The model under review builds one solid part; all positions refer to its coordinate system, in mm. Round coordinates to 2 decimals unless told otherwise and drop trailing zeros. Order: outer loops, then holes, each group sorted by start corner. A loop starts at its lowest first (then second) coordinate and runs counter-clockwise, first axis right, second up.
from build123d import *

# Parameters (mm, degrees)
F0_W     = 20
F0_H     = 20
F1_DEPTH = 240
F2_R     = 2.5
F3_DEPTH = 25
F4_R     = 2.5
F5_DEPTH = 25


with BuildPart() as f1:
    # F0 (on Front) → F1 (new body)
    with BuildSketch(Plane.XZ):
        with Locations((24.677172, -22.298429)):
            Rectangle(F0_W, F0_H)
    extrude(amount=F1_DEPTH)

    # F2 (on face) → F3 (cut)
    with BuildSketch(Plane.XY.offset(-12.298429)):
        with Locations((24.677172, -230)):
            Circle(F2_R)
    extrude(amount=-F3_DEPTH, mode=Mode.SUBTRACT)

    # F4 (on face) → F5 (cut)
    with BuildSketch(Plane.XY.offset(-12.298429)):
        with Locations((24.677172, -10)):
            Circle(F4_R)
    extrude(amount=-F5_DEPTH, mode=Mode.SUBTRACT)


solid = f1.part
(1) We need section A-A (y = -10). Give the boundary of the cut face in (x, z), and give its area (3 significant figures).
(2) The part is to be moulded in two halves that separate along Y. For faces 1 (the cylindrical face through (22.69, -11.52, -22.16)), 2 (the flat face through (25, -240, -22)), 3 (the flat face through (34.677, -118, -22)), say which applies: pulls with the +Y half, pulls with the -Y half, needs draft (parallel to the pull), parting line crosses it, or undercut.
(3) We need section B-B (x = 24.5). Give the boundary of the cut face in (y, z), and give its area (3 significant figures).
(4) Clearance check with flat-ended pins moving along their axes: P1, Ø3, axis at x = 24.68, y = -10, coming from the -Z side; P2, Ø5, axis at x = 21, z = -28, coming from the +Y side. State where each tip first meets the part, or that it passes through.
(5) To check wall thickness, follow L1, parallel to Y at x = 24.25, z = -22.25; L2, parallel to X at y = -230, z = -22.75; L3, parallel to Y at x = 26.75, z = -23.75. State the ranges of each line that lie inside material, in increasing order.
Verdict:
1. outline: (14.68, -32.3) - (22.18, -32.3) - (22.18, -12.3) - (14.68, -12.3) - close; (27.18, -32.3) - (34.68, -32.3) - (34.68, -12.3) - (27.18, -12.3) - close
1. area: 300 mm2
2. face 1: undercut
2. face 2: pulls with the -Y half
2. face 3: needs draft
3. outline: (-240, -32.3) - (-232.49, -32.3) - (-232.49, -12.3) - (-240, -12.3) - close; (-227.51, -32.3) - (-12.49, -32.3) - (-12.49, -12.3) - (-227.51, -12.3) - close; (-7.51, -32.3) - (0, -32.3) - (0, -12.3) - (-7.51, -12.3) - close
3. area: 4,600 mm2
4. P1: passes through
4. P2: stops at y = 0
5. L1: y = -240 to -232.46, -227.54 to -12.46, -7.54 to 0
5. L2: x = 14.68 to 22.18, 27.18 to 34.68
5. L3: y = -240 to -231.4, -228.6 to -11.4, -8.6 to 0
